from build123d import *

# Parameters (mm, degrees)
F0_W     = 136.1321210861
F0_H     = 95.5515094101
F0_W_2   = 118.5759752989
F0_H_2   = 78.5709768534
F1_DEPTH = 63.5
F2_W     = 80.5856101215
F2_H     = 25.0779332817
F3_DEPTH = 141.986
F4_R     = 6.7127269872
F5_DEPTH = 186.69


with BuildPart() as f1:
    # F0 (on Top) → F1 (new body)
    with BuildSketch(Plane.XY):
        with Locations((0.8634179831, 2.4463478476)):
            Rectangle(F0_W, F0_H)
        with Locations((1.007322222, 2.0146407187)):
            Rectangle(F0_W_2, F0_H_2, mode=Mode.SUBTRACT)
    extrude(amount=F1_DEPTH)

    # F2 (on face) → F3 (cut)
    with BuildSketch(Plane.XZ.offset(45.3294068575)):
        with Locations((-0.1439023763, 50.9610333592)):
            Rectangle(F2_W, F2_H)
    extrude(amount=-F3_DEPTH, mode=Mode.SUBTRACT)

    # F4 (on face) → F5 (cut)
    with BuildSketch(Plane(origin=(-67.20264256, 0, 0), x_dir=(0, -1, 0), z_dir=(-1, 0, 0))):
        with Locations((-3.597572213, 33.8171757758)):
            Circle(F4_R)
    extrude(amount=-F5_DEPTH, mode=Mode.SUBTRACT)


solid = f1.part
Can you work these out from the model? Positions are in its coordinate system, mm. A direction names the side the tool comes from. Coordinates: 2 decimals unless noted, no trailing zeros. Write each loop counter-clockwise with the first axis right and the second up, starting at its lowest first coordinate (ties: lowest second). Pieces come first, ordered by that corner, then holes. Notation, with made-up numbers: (12, -12) - (42, -12) arc R24 cw to (42, 4) - close; hole circle Ø4 at (40, -35). An arc over 180 degrees is marked (long way). Return JSON: item names as keys, results as strings. Group by question number.
Item 1: Please list where these lines run through material, in increasing order: probe 1 along X at (y, z) = (7.5, 19.5); probe 2 along Y at (x, z) = (26, 10.5); probe 3 along X at (y, z) = (-41, 44).
Item 2: We'd pull the mould along X, two halves only. Please class faces 4 (the face through (-1, 46, 38.422)), 5 (the face through (64.552, 5.053, 27.264)), 6 (the face through (68.929, 2, 24)): pulls with the +X half, pulls with the -X half, needs draft (parallel to the pull), parting line crosses it, or undercut.
Item 3: I'm going to push a flat-ended pin straight in: pin 1 Ø9 at (x, y) = (3.5, -40) entering from +Z. Where does the tip first touch, or does it pass through?
Item 4: If we section it at C-C (x = -51.5): Write out the boundary of the cut face in (y, z), then the cut area to 3 significant figures.
Item 5: If we section it at B-B (y = 39.5): Write out the boundary of the cut face in (x, z).
Item 6: If we section it at D-D (y = 0): Write out the boundary of the cut face in (x, z).
Item 7: If we section it at A-A (z = 51): Write out the boundary of the cut face in (x, y).
Item 8: Which directions (+Z, -Z, +X, -X, +Y, -Y) give clear straight access to the entire face, cutting with the end or side of a thin tool? Please do faces 1 (the face through (0, -45.329, 24)), 2 (the face through (40.149, -41, 51)), 3 (the face through (-58.281, 1, 24)).
Return value:
{
 "1": {"probe 1": "x = -67.2 to -58.28, 60.3 to 68.93", "probe 2": "y = -45.33 to -37.27, 41.3 to 50.22", "probe 3": "x = -67.2 to -40.44, 40.15 to 68.93"},
 "2": {"face 4": "undercut", "face 5": "needs draft", "face 6": "pulls with the +X half"},
 "3": {"pin 1": "stops at z = 38.42"},
 "4": {"outline": "(-45.33, 0) - (-37.27, 0) - (-37.27, 63.5) - (-45.33, 63.5) - close; (41.3, 0) - (50.22, 0) - (50.22, 63.5) - (41.3, 63.5) - close", "area": "1,080 mm^2"},
 "5": {"outline": "(-67.2, 0) - (-58.28, 0) - (-58.28, 63.5) - (-67.2, 63.5) - close; (60.3, 0) - (68.93, 0) - (68.93, 63.5) - (60.3, 63.5) - close"},
 "6": {"outline": "(-67.2, 0) - (-58.28, 0) - (-58.28, 28.15) - (-67.2, 28.15) - close; (-67.2, 39.48) - (-58.28, 39.48) - (-58.28, 63.5) - (-67.2, 63.5) - close; (60.3, 0) - (68.93, 0) - (68.93, 28.15) - (60.3, 28.15) - close; (60.3, 39.48) - (68.93, 39.48) - (68.93, 63.5) - (60.3, 63.5) - close"},
 "7": {"outline": "(-67.2, -45.33) - (-40.44, -45.33) - (-40.44, -37.27) - (-58.28, -37.27) - (-58.28, 41.3) - (-40.44, 41.3) - (-40.44, 50.22) - (-67.2, 50.22) - close; (40.15, -45.33) - (68.93, -45.33) - (68.93, 50.22) - (40.15, 50.22) - (40.15, 41.3) - (60.3, 41.3) - (60.3, -37.27) - (40.15, -37.27) - close"},
 "8": {"face 1": "+Z, -Z, +X, -X, -Y", "face 2": "+Z, +Y, -Y", "face 3": "+Z, -Z"}
}
